Study the drawing (mm; zero at the part's minimum x, y, z) and answer. A direction names the side the tool comes from. Give positions to 0.01 mm unless a question says otherwise; leave off trailing zeros. Write each loop counter-clockwise with the first axis right and the second up, starting at its lowest first coordinate (ties: lowest second). Pieces come first, ordered by that corner, then holes. Notation, with made-up numbers: (72, 28) - (106, 28) arc R9 ccw to (106, 40) - close; hole circle Ø1 at (-24.5, 20). An arc over 180 degrees is marked (long way). Return JSON: item names as keys, results as strings.
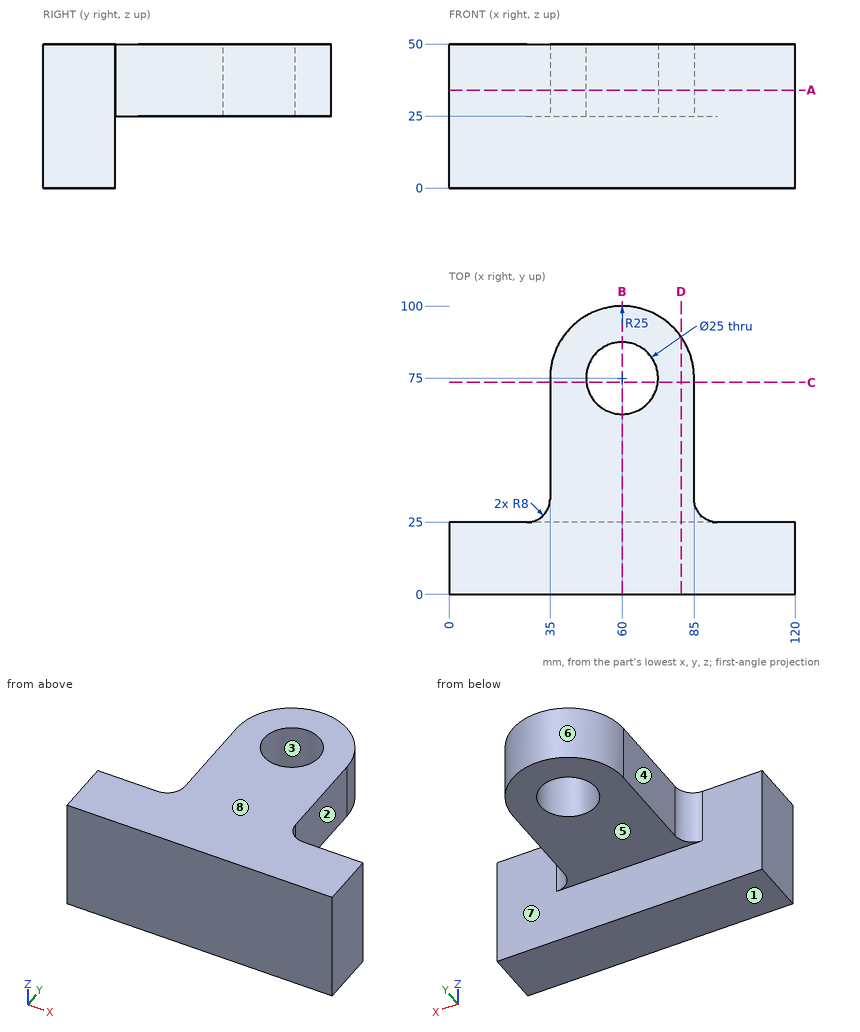
Item 1: A cutting plane is placed at C-C on y = 73.5. Determine the outline of the cut face in (x, z).
Answer below:
{"outline": "(35, 25) - (47.59, 25) - (47.59, 50) - (35, 50) - close; (72.41, 25) - (85, 25) - (85, 50) - (72.41, 50) - close"}
Item 2: A cutting plane is placed at A-A on z = 34. Determine the outline of the cut face in (x, y).
Answer below:
{"outline": "(0, 0) - (120, 0) - (120, 25) - (93, 25) arc R8 cw to (85, 33) - (85, 75) arc R25 ccw to (35, 75) - (35, 33) arc R8 cw to (27, 25) - (0, 25) - close; hole circle Ø25 at (60, 75)"}
Item 3: Consider L1, parallel to Y at x = 60, z = 41.25; L2, parallel to Z at x = 48, y = 38; L3, parallel to Y at x = 13, z = 24. Determine where each line is inside the solid, lowest interval first.
Answer below:
{"L1": "y = 0 to 62.5, 87.5 to 100", "L2": "z = 25 to 50", "L3": "y = 0 to 25"}
Item 4: For the marked faces 4, 5, 6, 7 and 8, determine the directions among +Z, -Z, +X, -X, +Y, -Y from which every point of the face is accessible in a straight line to the end or side of a thin tool.
Answer below:
{"face 4": "+Z, -Z, -X, +Y", "face 5": "-Z, +X, -X, +Y", "face 6": "+Z, -Z, +Y", "face 7": "-Z, +Y", "face 8": "+Z, +X, -X, +Y, -Y"}
Item 5: Flat-ended cylindrical pins translate along their axes: P1, Ø20, axis at x = 60, y = 75, coming from the +Z side; P2, Ø6, axis at x = 15.5, z = 8.5, coming from the +Y side; P3, Ø4, axis at x = 52.5, y = 85, coming from the -Z side; P4, Ø6, axis at x = 31, y = 27, coming from the -Z side. Find the tip coordinate at first contact, or state that the pin passes through.
Answer below:
{"P1": "passes through", "P2": "stops at y = 25", "P3": "stops at z = 25", "P4": "stops at z = 0"}
Item 6: The mould has two halves that part along X. Classify the marked faces 1, 2 and 3: +X half, -X half, draft (parallel to the pull), parting line (faces both ways), or undercut.
Answer below:
{"face 1": "draft", "face 2": "+X half", "face 3": "undercut"}
Item 7: A cutting plane is placed at B-B on x = 60. Determine the outline of the cut face in (y, z), then the cut area to 3 significant figures.
Answer below:
{"outline": "(0, 0) - (25, 0) - (25, 25) - (62.5, 25) - (62.5, 50) - (0, 50) - close; (87.5, 25) - (100, 25) - (100, 50) - (87.5, 50) - close", "area": "2,500 mm²"}
Item 8: A cutting plane is placed at D-D on x = 80.5. Determine the outline of the cut face in (y, z).
Answer below:
{"outline": "(0, 0) - (25, 0) - (25, 25) - (89.31, 25) - (89.31, 50) - (0, 50) - close"}
